Read the model definition and answer for the solid it produces. Units are mm, in the model's axes. Face numbers are marked on the shaded views. A direction names the side the tool comes from. Coordinates: 2 decimals unless noted, no trailing zeros. Write each loop counter-clockwise with the first axis right and the second up, starting at its lowest first coordinate (ties: lowest second). Pieces come first, ordered by that corner, then holes.
(1) Given pin 1 (4 mm diameter, centred on x = 11, z = 3, fed in from -Y), flat-ended and moving along its own axis, determine where the tip first touches the part or whether it passes through.
(2) Find the intervals of material crossed by probe 1 along X at (y, z) = (11.5, 3); probe 2 along Y at (x, z) = (29.5, -5); probe 3 along X at (y, z) = (20, -11.5), in increasing order.
(3) Section C-C on x = 10.5 is taken. Write down the section's boundary in (y, z) (3 decimals), then the cut area to 3 significant figures.
(4) Section A-A on y = 19 is taken. Write down the section's boundary in (x, z), then the cut area to 3 significant figures.
(5) Section D-D on z = -13.25 is taken. Write down the section's boundary in (x, y), then the cut area to 3 significant figures.
(6) Section B-B on z = 0.5 is taken. Write down the section's boundary in (x, y) (3 decimals).
(7) Which of the six approach directions +Z, -Z, +X, -X, +Y, -Y give full straight-line access (tool end or side, diameter ignored) to the marked faces 1, 2 and 3?
(8) The mould has two halves that part along X. Classify the marked faces 4, 5, 6 and 7: +X half, -X half, draft (parallel to the pull), parting line (faces both ways), or undercut.
from build123d import *

# Parameters (mm, degrees)
F0_W     = 35
F0_H     = 25
F0_W_2   = 9.25
F0_H_2   = 14.35
F1_DEPTH = 5.5
F3_DEPTH = 15
F4_SIZE  = 0.8


with BuildPart() as f1:
    # F0 (on Top) → F1 (new body)
    with BuildSketch(Plane.XY):
        with Locations((17.5, 12.5)):
            Rectangle(F0_W, F0_H)
        with Locations((8.731327, 12.5)):
            Rectangle(F0_W_2, F0_H_2, mode=Mode.SUBTRACT)
        with Locations((26.268673, 12.5)):
            Rectangle(F0_W_2, F0_H_2, mode=Mode.SUBTRACT)
    extrude(amount=F1_DEPTH)

    # F2 (on face) → F3 (join)
    with BuildSketch(Plane(origin=(0, 0, 0), x_dir=(1, 0, 0), z_dir=(0, 0, -1))):
        Polygon((35, 0), (0, 0), (0, -7.563511), (1.5, -7.563511), (1.5, -1.5), (33.5, -1.5), (33.5, -7.563511), (35, -7.563511), align=None)
        Polygon((1.5, -17.436489), (0, -17.436489), (0, -25), (35, -25), (35, -17.436489), (33.5, -17.436489), (33.5, -23.5), (1.5, -23.5), align=None)
    extrude(amount=F3_DEPTH)

    # F4
    f4_edges = [f1.edges().sort_by_distance(p)[0] for p in [
        (8.731327, 19.675, 5.5),
        (8.731327, 5.325, 5.5),
        (26.268673, 19.675, 5.5),
        (26.268673, 5.325, 5.5),
    ]]
    chamfer(f4_edges, length=F4_SIZE)


solid = f1.part
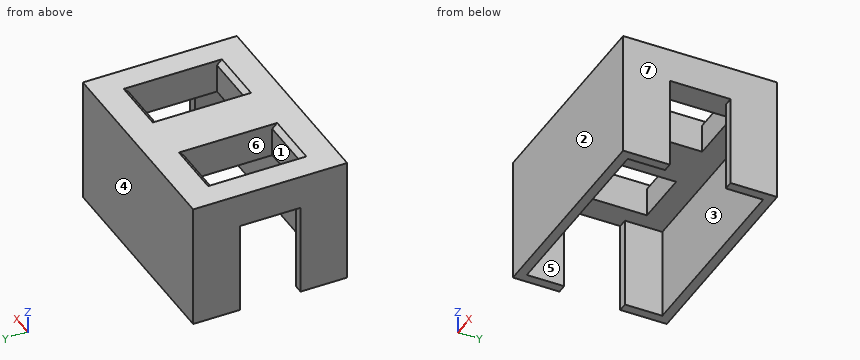
Response:
1. pin 1: stops at y = 0
2. probe 1: x = 0 to 4.11, 13.36 to 21.64, 30.89 to 35
2. probe 2: y = 0 to 1.5, 23.5 to 25
2. probe 3: x = 0 to 1.5, 33.5 to 35
3. outline: (0, -15) - (1.5, -15) - (1.5, 0) - (5.325, 0) - (5.325, 4.7) - (4.525, 5.5) - (0, 5.5) - close; (19.675, 0) - (23.5, 0) - (23.5, -15) - (25, -15) - (25, 5.5) - (20.475, 5.5) - (19.675, 4.7) - close
3. area: 103 mm2
4. outline: (0, -15) - (1.5, -15) - (1.5, 0) - (4.11, 0) - (4.11, 5.5) - (0, 5.5) - close; (13.36, 0) - (21.64, 0) - (21.64, 5.5) - (13.36, 5.5) - close; (30.89, 0) - (33.5, 0) - (33.5, -15) - (35, -15) - (35, 5.5) - (30.89, 5.5) - close
4. area: 136 mm2
5. outline: (0, 0) - (35, 0) - (35, 7.56) - (33.5, 7.56) - (33.5, 1.5) - (1.5, 1.5) - (1.5, 7.56) - (0, 7.56) - close; (0, 17.44) - (1.5, 17.44) - (1.5, 23.5) - (33.5, 23.5) - (33.5, 17.44) - (35, 17.44) - (35, 25) - (0, 25) - close
5. area: 141 mm2
6. outline: (0, 0) - (35, 0) - (35, 25) - (0, 25) - close; hole (4.106, 5.325) - (13.356, 5.325) - (13.356, 19.675) - (4.106, 19.675) - close; hole (21.644, 5.325) - (30.894, 5.325) - (30.894, 19.675) - (21.644, 19.675) - close
7. face 1: +Z, -Z
7. face 2: +Z, -Z, +X, -X, -Y
7. face 3: -Z
8. face 4: draft
8. face 5: undercut
8. face 6: undercut
8. face 7: +X half
